The model under review builds one solid part; all positions refer to its coordinate system, in mm. Face numbers are marked on the shaded views. Coordinates: 2 decimals unless noted, no trailing zeros. Loops run counter-clockwise (first coordinate to the right, second up) from the corner with the lowest first, then second, coordinate; pieces in that order, holes last. Notation, with made-up numbers: M -12,-2 L 38,-2 A18 cw 38,11 Z; hole C 16,12 d3. An arc over 180 degrees is marked long. Return JSON: item names as keys, results as strings.
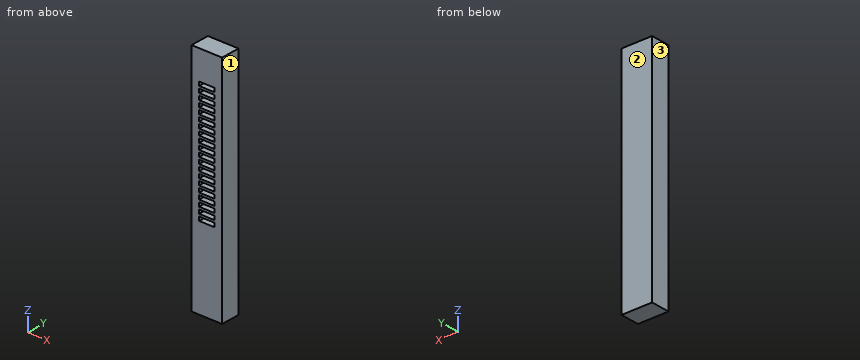
```python
from build123d import *

# Parameters (mm, degrees)
F0_W     = 200
F0_H     = 1500
F0_W_2   = 100
F0_H_2   = 25
F1_DEPTH = 20
F2_W     = 200
F2_H     = 1500
F2_W_2   = 160
F2_H_2   = 1450
F3_DEPTH = 60
F4_W     = 200
F4_H     = 1500
F5_DEPTH = 20
F6_DEPTH = 25


with BuildPart() as f1:
    # F0 (on Front) → F1 (new body)
    with BuildSketch(Plane.XZ):
        Rectangle(F0_W, F0_H)
        with Locations((0.320368, -209.9976)):
            Rectangle(F0_W_2, F0_H_2, mode=Mode.SUBTRACT)
        with Locations((0.320368, -169.9976)):
            Rectangle(F0_W_2, F0_H_2, mode=Mode.SUBTRACT)
        with Locations((0.052069, -130)):
            Rectangle(F0_W_2, F0_H_2, mode=Mode.SUBTRACT)
        with Locations((0, -90)):
            Rectangle(F0_W_2, F0_H_2, mode=Mode.SUBTRACT)
        with Locations((0, -50)):
            Rectangle(F0_W_2, F0_H_2, mode=Mode.SUBTRACT)
        with Locations((0, -10)):
            Rectangle(F0_W_2, F0_H_2, mode=Mode.SUBTRACT)
        with Locations((0, 30)):
            Rectangle(F0_W_2, F0_H_2, mode=Mode.SUBTRACT)
        with Locations((0, 70)):
            Rectangle(F0_W_2, F0_H_2, mode=Mode.SUBTRACT)
        with Locations((0, 110)):
            Rectangle(F0_W_2, F0_H_2, mode=Mode.SUBTRACT)
        with Locations((0, 150)):
            Rectangle(F0_W_2, F0_H_2, mode=Mode.SUBTRACT)
        with Locations((0, 190)):
            Rectangle(F0_W_2, F0_H_2, mode=Mode.SUBTRACT)
        with Locations((0, 230)):
            Rectangle(F0_W_2, F0_H_2, mode=Mode.SUBTRACT)
        with Locations((0, 270)):
            Rectangle(F0_W_2, F0_H_2, mode=Mode.SUBTRACT)
        with Locations((0, 310)):
            Rectangle(F0_W_2, F0_H_2, mode=Mode.SUBTRACT)
        with Locations((0, 350)):
            Rectangle(F0_W_2, F0_H_2, mode=Mode.SUBTRACT)
        with Locations((0, 390)):
            Rectangle(F0_W_2, F0_H_2, mode=Mode.SUBTRACT)
        with Locations((0, 430)):
            Rectangle(F0_W_2, F0_H_2, mode=Mode.SUBTRACT)
        with Locations((0, 470)):
            Rectangle(F0_W_2, F0_H_2, mode=Mode.SUBTRACT)
        with Locations((0, 510)):
            Rectangle(F0_W_2, F0_H_2, mode=Mode.SUBTRACT)
        with Locations((0, 550)):
            Rectangle(F0_W_2, F0_H_2, mode=Mode.SUBTRACT)
    extrude(amount=-F1_DEPTH)

    # F2 (on face) → F3 (join)
    with BuildSketch(Plane(origin=(0, 20, 0), x_dir=(-1, 0, 0), z_dir=(0, 1, 0))):
        Rectangle(F2_W, F2_H)
        Rectangle(F2_W_2, F2_H_2, mode=Mode.SUBTRACT)
    extrude(amount=F3_DEPTH)

    # F4 (on face) → F5 (join)
    with BuildSketch(Plane(origin=(0, 80, 0), x_dir=(-1, 0, 0), z_dir=(0, 1, 0))):
        Rectangle(F4_W, F4_H)
    extrude(amount=F5_DEPTH)

    # F0 (on Front) → F6 (join)
    with BuildSketch(Plane.XZ):
        Rectangle(F0_W, F0_H)
        with Locations((0.320368, -209.9976)):
            Rectangle(F0_W_2, F0_H_2, mode=Mode.SUBTRACT)
        with Locations((0.320368, -169.9976)):
            Rectangle(F0_W_2, F0_H_2, mode=Mode.SUBTRACT)
        with Locations((0.052069, -130)):
            Rectangle(F0_W_2, F0_H_2, mode=Mode.SUBTRACT)
        with Locations((0, -90)):
            Rectangle(F0_W_2, F0_H_2, mode=Mode.SUBTRACT)
        with Locations((0, -50)):
            Rectangle(F0_W_2, F0_H_2, mode=Mode.SUBTRACT)
        with Locations((0, -10)):
            Rectangle(F0_W_2, F0_H_2, mode=Mode.SUBTRACT)
        with Locations((0, 30)):
            Rectangle(F0_W_2, F0_H_2, mode=Mode.SUBTRACT)
        with Locations((0, 70)):
            Rectangle(F0_W_2, F0_H_2, mode=Mode.SUBTRACT)
        with Locations((0, 110)):
            Rectangle(F0_W_2, F0_H_2, mode=Mode.SUBTRACT)
        with Locations((0, 150)):
            Rectangle(F0_W_2, F0_H_2, mode=Mode.SUBTRACT)
        with Locations((0, 190)):
            Rectangle(F0_W_2, F0_H_2, mode=Mode.SUBTRACT)
        with Locations((0, 230)):
            Rectangle(F0_W_2, F0_H_2, mode=Mode.SUBTRACT)
        with Locations((0, 270)):
            Rectangle(F0_W_2, F0_H_2, mode=Mode.SUBTRACT)
        with Locations((0, 310)):
            Rectangle(F0_W_2, F0_H_2, mode=Mode.SUBTRACT)
        with Locations((0, 350)):
            Rectangle(F0_W_2, F0_H_2, mode=Mode.SUBTRACT)
        with Locations((0, 390)):
            Rectangle(F0_W_2, F0_H_2, mode=Mode.SUBTRACT)
        with Locations((0, 430)):
            Rectangle(F0_W_2, F0_H_2, mode=Mode.SUBTRACT)
        with Locations((0, 470)):
            Rectangle(F0_W_2, F0_H_2, mode=Mode.SUBTRACT)
        with Locations((0, 510)):
            Rectangle(F0_W_2, F0_H_2, mode=Mode.SUBTRACT)
        with Locations((0, 550)):
            Rectangle(F0_W_2, F0_H_2, mode=Mode.SUBTRACT)
    extrude(amount=F6_DEPTH)


solid = f1.part
```
1. Add section A-A on z = 632. Give the boundary of the cut face in (x, y).
Check values:
{"outline": "M -100,-25 L 100,-25 L 100,100 L -100,100 Z; hole M -80,20 L 80,20 L 80,80 L -80,80 Z"}
2. The part is to be moulded in two halves that separate along X. For the marked faces 1, 2 and 3, say which applies: released by +X, released by -X, zero draft, split by the parting line, or undercut.
Check values:
{"face 1": "released by +X", "face 2": "zero draft", "face 3": "released by -X"}
3. Add section B-B on y = 55.5. Give the boundary of the cut face in (x, z), plus the area to 3 significant figures.
Check values:
{"outline": "M -100,-750 L 100,-750 L 100,750 L -100,750 Z; hole M -80,-725 L 80,-725 L 80,725 L -80,725 Z", "area": "68,000 mm²"}
4. To check wall thickness, follow line 1 (Y direction, x = 73.5, z = -374); line 2 (X direction, y = 39.5, z = -642); line 3 (Z direction, x = 67, y = 22.5). State the ranges of each line that lie inside material, in increasing order.
Check values:
{"line 1": "-25 to 20, 80 to 100", "line 2": "-100 to -80, 80 to 100", "line 3": "-750 to -725, 725 to 750"}
5. Add section C-C on x = 35.5. State how many separate pieces and enclosed holes the cut face has, plus the area to 3 significant figures.
Check values:
{"separate pieces": "20", "enclosed holes": "0", "area": "78,000 mm²"}
